from build123d import *

# Parameters (mm, degrees)
EXTRUDE_1_DEPTH      = 10
SKETCH_7_R           = 1.55
CUT_EXTRUDE_1_DEPTH  = 47.544157215
CUT_EXTRUDE_2_DEPTH  = 18.5
SKETCH_19_W          = 126.714157214
SKETCH_19_H          = 0.99604336
CUT_EXTRUDE_14_DEPTH = 51.044157215
SKETCH_23_R          = 1.575
CUT_EXTRUDE_16_DEPTH = 10
SKETCH_24_R          = 3.35
CUT_EXTRUDE_17_DEPTH = 2.5


with BuildPart() as part:
    # 草图1 → 凸台-拉伸1 (new body)
    with BuildSketch(Plane.XY):
        Polygon((-3.188712924, 13.052848472), (33.811287076, 13.052848472), (33.811287076, 7.052848472), (15.60198174, 7.052848472), (11.74198174, 7.052848472), (-12.185815886, -36.991308743), (-14.185815886, -36.991308743), (-29.545791531, -36.991308743), (-27.045791531, -31.991308743), (-17.548712924, -31.991308743), align=None)
    extrude_1 = extrude(amount=EXTRUDE_1_DEPTH)

    # 镜向1: 凸台-拉伸1 across plane
    add(extrude_1.mirror(Plane(origin=(33.811287076, 13.052848472, 10), x_dir=(0, 0, 1), z_dir=(-1, 0, 0))))

    # 草图5 → 切除-旋转7 (revolve, cut)
    with BuildSketch(Plane.XY.offset(5)):
        Polygon((7.961287076, 13.052848472), (7.961287076, 10.552848472), (7.161287076, 10.552848472), (7.161287076, 9.552848472), (6.361287076, 9.552848472), (4.811287076, 9.552848472), (4.811287076, 13.052848472), align=None)
    cut_revolve_7 = revolve(axis=Axis((4.811287076, 9.552848472, 5), (0, 1, 0)), mode=Mode.SUBTRACT)

    # 草图7 → 切除-拉伸1 (cut, through all)
    with BuildSketch(Plane(origin=(0, 9.552848472, 0), x_dir=(1, 0, 0), z_dir=(0, 1, 0))):
        with Locations((4.811287076, -5)):
            Circle(SKETCH_7_R)
    cut_extrude_1 = extrude(amount=-CUT_EXTRUDE_1_DEPTH, mode=Mode.SUBTRACT)

    # 草图8 → 切除-拉伸2 (cut)
    with BuildSketch(Plane(origin=(0, -11.947151528, 0), x_dir=(1, 0, 0), z_dir=(0, 1, 0))):
        Polygon((8.333123718, -5), (6.572205397, -1.95), (3.050368755, -1.95), (1.289450434, -5), (3.050368755, -8.05), (6.572205397, -8.05), align=None)
    cut_extrude_2 = extrude(amount=CUT_EXTRUDE_2_DEPTH, mode=Mode.SUBTRACT)

    # 草图19 → 切除-拉伸14 (cut, through all)
    with BuildSketch(Plane(origin=(0, 13.052848472, 0), x_dir=(1, 0, 0), z_dir=(0, 1, 0))):
        with Locations((33.811287076, -9.50197832)):
            Rectangle(SKETCH_19_W, SKETCH_19_H)
    extrude(amount=-CUT_EXTRUDE_14_DEPTH, mode=Mode.SUBTRACT)

    # 草图23 → 切除-拉伸16 (cut)
    with BuildSketch(Plane(origin=(0, -31.991308743, 0), x_dir=(1, 0, 0), z_dir=(0, 1, 0))):
        with Locations((-22.548712924, -5)):
            Circle(SKETCH_23_R)
    cut_extrude_16 = extrude(amount=-CUT_EXTRUDE_16_DEPTH, mode=Mode.SUBTRACT)

    # 草图24 → 切除-拉伸17 (cut)
    with BuildSketch(Plane(origin=(0, -31.991308743, 0), x_dir=(1, 0, 0), z_dir=(0, 1, 0))):
        with Locations((-22.548712924, -5)):
            Circle(SKETCH_24_R)
    cut_extrude_17 = extrude(amount=-CUT_EXTRUDE_17_DEPTH, mode=Mode.SUBTRACT)

    # 镜向3: 切除-旋转7, 切除-拉伸1, 切除-拉伸2, 切除-拉伸16, 切除-拉伸17 across plane
    add(cut_revolve_7.mirror(Plane(origin=(33.811287076, 0, 0), x_dir=(0, 0, 1), z_dir=(1, 0, 0))), mode=Mode.SUBTRACT)
    add(cut_extrude_1.mirror(Plane(origin=(33.811287076, 0, 0), x_dir=(0, 0, 1), z_dir=(1, 0, 0))), mode=Mode.SUBTRACT)
    add(cut_extrude_2.mirror(Plane(origin=(33.811287076, 0, 0), x_dir=(0, 0, 1), z_dir=(1, 0, 0))), mode=Mode.SUBTRACT)
    add(cut_extrude_16.mirror(Plane(origin=(33.811287076, 0, 0), x_dir=(0, 0, 1), z_dir=(1, 0, 0))), mode=Mode.SUBTRACT)
    add(cut_extrude_17.mirror(Plane(origin=(33.811287076, 0, 0), x_dir=(0, 0, 1), z_dir=(1, 0, 0))), mode=Mode.SUBTRACT)


solid = part.part
Input: part model. Units: mm. Frame: model coordinates. A direction names the side the tool comes from. Round coordinates to 2 decimals unless told otherwise and drop trailing zeros. Loops run counter-clockwise (first coordinate to the right, second up) from the corner with the lowest first, then second, coordinate; pieces in that order, holes last. Notation, with made-up numbers: (19.25, 87.25) -> (64.25, 87.25) arc R9 ccw to (64.25, 104.25) -> close; hole circle Ø2 at (66, 29.25). An arc over 180 degrees is marked (long way). Answer as a JSON object with one key per item and string values. Group by question number.
1) Ray query, L1, parallel to X at y = 5, z = 3; L2, parallel to X at y = -33.25, z = 5; L3, parallel to X at y = 9.9, z = 5. Return the intervals inside material, ascending.
2) Section query C-C on y = -4.5. Output: boundary loops of the cut face in (x, z), plus the area to 3 significant figures.
3) Draft query along X for faces 1 (the flat face through (88, -31.991, 2)), 2 (the flat face through (60.182, 2.983, 6.546)), 3 (the flat face through (-10.469, -9.785, 4.439)). Return one class per face: +X half, -X half, draft (parallel to the pull), parting line (faces both ways), or undercut.
4) Reachability of faces 4 (the flat face through (7.465, 2.983, 3.496)), 5 (the flat face through (34, 13.053, 4)), 6 (the flat face through (-21, -34.491, 6)), 7 (the flat face through (67.7, -14.7, 4.4)) from +Z, -Z, +X, -X, +Y, -Y: full face, straight path, thin tool, end or side. Return the list, or none.
5) Section query B-B on x = 26.5. Output: boundary loops of the cut face in (y, z).
6) Section query A-A on y = -27.5. Output: boundary loops of the cut face in (x, z).
7) Pin query (flat end, axial travel): pin 1 (3 mm diameter, centred on x = 90.17, z = 5, fed in from -Y); pin 2 (5 mm diameter, centred on x = 1.5, z = 6.5, fed in from -Y); pin 3 (5 mm diameter, centred on y = 4, z = 7, fed in from -X); pin 4 (5 mm diameter, centred on x = 39, z = 2.5, fed in from -Y). Return the tip coordinate at first contact, or that it passes through.
Reply:
{
 "1": {"L1": "x = -5.76 to 2.44, 7.18 to 10.63, 57 to 60.44, 65.18 to 73.38", "L2": "x = -27.68 to -25.9, -19.2 to -10.15, 77.78 to 86.82, 93.52 to 95.3", "L3": "x = -4.19 to 2.46, 7.16 to 60.46, 65.16 to 71.82"},
 "2": {"outline": "(-8.78, 0) -> (5.47, 0) -> (5.47, 1.95) -> (3.05, 1.95) -> (1.29, 5) -> (3.05, 8.05) -> (5.47, 8.05) -> (5.47, 9) -> (-8.78, 9) -> close; (62.16, 0) -> (76.41, 0) -> (76.41, 9) -> (62.16, 9) -> (62.16, 8.05) -> (64.57, 8.05) -> (66.33, 5) -> (64.57, 1.95) -> (62.16, 1.95) -> close", "area": "216 mm2"},
 "3": {"face 1": "draft", "face 2": "undercut", "face 3": "-X half"},
 "4": {"face 4": "-Y", "face 5": "+Z, -Z, +X, -X, +Y", "face 6": "+Y", "face 7": "+Z, -Z, -Y"},
 "5": {"outline": "(7.05, 0) -> (13.05, 0) -> (13.05, 9) -> (7.05, 9) -> close"},
 "6": {"outline": "(-16.12, 0) -> (-7.03, 0) -> (-7.03, 9) -> (-16.12, 9) -> close; (74.65, 0) -> (83.74, 0) -> (83.74, 9) -> (74.65, 9) -> close"},
 "7": {"pin 1": "passes through", "pin 2": "stops at y = -16.4", "pin 3": "stops at x = -6.87", "pin 4": "stops at y = 7.05"}
}
